```python
from build123d import *

# Parameters (mm, degrees)
SKETCH_R   = 2
SKETCH_R_2 = 1.5
PAD_DEPTH  = 2
FILLET_R   = 4


with BuildPart() as part:
    # Sketch → Pad (new body)
    with BuildSketch(Plane.XY):
        Polygon((-46, -4), (46, -4), (46, 4), (0, 14), (-46, 4), align=None)
        with Locations((-42, 0)):
            Circle(SKETCH_R, mode=Mode.SUBTRACT)
        with Locations((42, 0)):
            Circle(SKETCH_R, mode=Mode.SUBTRACT)
        with Locations((0, 10)):
            Circle(SKETCH_R_2, mode=Mode.SUBTRACT)
    extrude(amount=PAD_DEPTH)

    # Fillet
    fillet_edges = [part.edges().sort_by_distance(p)[0] for p in [
        (46, -4, 1),
        (46, 4, 1),
        (-46, -4, 1),
        (-46, 4, 1),
        (0, 14, 1),
    ]]
    fillet(fillet_edges, radius=FILLET_R)


solid = part.part
```
For this review, take the finished solid that the model builds, in its own axes (mm). Coordinates: 2 decimals unless noted, no trailing zeros. Write each loop counter-clockwise with the first axis right and the second up, starting at its lowest first coordinate (ties: lowest second). Pieces come first, ordered by that corner, then holes.
(1) Add section B-B on x = 0. Give the boundary of the cut face in (y, z), then the cut area to 3 significant figures.
(2) Add section C-C on z = 1.2. Give the boundary of the cut face in (x, y), then the cut area to 3 significant figures.
(3) The part is to be moulded in two halves that separate along X. For faces 1 (the face through (44.797, -2.859, 1.014)), 2 (the face through (40, 0, 1)), 3 (the face through (-1, -4, 1)), 4 (the face through (-0.325, 8.536, 0.986)), say which applies: +X half, -X half, draft (parallel to the pull), parting line (faces both ways), or undercut.
(4) Add section A-A on y = 10. Give the boundary of the cut face in (x, z).
(5) Add section D-D on x = -33. Give the boundary of the cut face in (y, z).
(6) Wall thickness on probe 1 along X at (y, z) = (-0.5, 1); probe 2 along Y at (x, z) = (-11, 1.6); probe 3 along X at (y, z) = (3.75, 0.8): over which ranges is each line inside the solid? List them lowest first.
Answer sheet:
1. outline: (-4, 0) - (8.5, 0) - (8.5, 2) - (-4, 2) - close; (11.5, 0) - (13.91, 0) - (13.91, 2) - (11.5, 2) - close
1. area: 29.8 mm2
2. outline: (-46, 0) arc R4 ccw to (-42, -4) - (42, -4) arc R4 ccw to (46, 0) - (46, 0.78) arc R4 ccw to (42.85, 4.68) - (0.85, 13.82) arc R4 ccw to (-0.85, 13.82) - (-42.85, 4.68) arc R4 ccw to (-46, 0.78) - close; hole circle Ø4 at (-42, 0); hole circle Ø3 at (0, 10); hole circle Ø4 at (42, 0)
2. area: 1,150 mm2
3. face 1: +X half
3. face 2: undercut
3. face 3: draft
3. face 4: undercut
4. outline: (-18.4, 0) - (-1.5, 0) - (-1.5, 2) - (-18.4, 2) - close; (1.5, 0) - (18.4, 0) - (18.4, 2) - (1.5, 2) - close
5. outline: (-4, 0) - (6.83, 0) - (6.83, 2) - (-4, 2) - close
6. probe 1: x = -45.97 to -43.94, -40.06 to 40.06, 43.94 to 45.97
6. probe 2: y = -4 to 11.61
6. probe 3: x = -44.68 to 44.68
